```python
from build123d import *

# Parameters (mm, degrees)
PAD_DEPTH   = 25
FILLET_R    = 1.5
FILLET001_R = 1.5


with BuildPart() as part:
    # Sketch → Pad (new body)
    with BuildSketch(Plane.XY):
        with BuildLine():
            Line((0, 0), (0, -45))
            ThreePointArc((-4, -41), (-2.828427, -43.828427), (0, -45))
            Line((-4, -41), (-4, -37))
            ThreePointArc((-4, -37), (-5.171573, -34.171573), (-8, -33))
            Line((-8, -33), (-36, -33))
            ThreePointArc((-40, -29), (-38.828427, -31.828427), (-36, -33))
            Line((-40, -29), (-40, 0))
            ThreePointArc((-36, 0), (-38, 2), (-40, 0))
            Line((-36, 0), (-36, -25))
            ThreePointArc((-36, -25), (-34.828427, -27.828427), (-32, -29))
            Line((-32, -29), (-8, -29))
            ThreePointArc((-8, -29), (-5.171573, -27.828427), (-4, -25))
            Line((-4, -25), (-4, 0))
            ThreePointArc((0, 4), (-2.828427, 2.828427), (-4, 0))
            Line((0, 4), (36, 4))
            ThreePointArc((40, 0), (38.828427, 2.828427), (36, 4))
            Line((40, 0), (0, 0))
        make_face()
    extrude(amount=PAD_DEPTH)

    # Fillet
    fillet_edges = [part.edges().sort_by_distance(p)[0] for p in [
        (-2.828427, -43.828427, 25),
        (-4, -39, 25),
        (-5.171573, -34.171573, 25),
        (-22, -33, 25),
        (-38.828427, -31.828427, 25),
        (-40, -14.5, 25),
        (-38, 2, 25),
        (-36, -12.5, 25),
        (-34.828427, -27.828427, 25),
        (-20, -29, 25),
        (-5.171573, -27.828427, 25),
        (-4, -12.5, 25),
        (-2.828427, 2.828427, 25),
        (18, 4, 25),
        (38.828427, 2.828427, 25),
    ]]
    fillet(fillet_edges, radius=FILLET_R)

    # Fillet001
    fillet001_edges = [part.edges().sort_by_distance(p)[0] for p in [
        (38.828427, 2.828427, 0),
        (18, 4, 0),
        (-2.828427, 2.828427, 0),
        (-4, -12.5, 0),
        (-5.171573, -27.828427, 0),
        (-20, -29, 0),
        (-34.828427, -27.828427, 0),
        (-36, -12.5, 0),
        (-38, 2, 0),
        (-40, -14.5, 0),
        (-38.828427, -31.828427, 0),
        (-22, -33, 0),
        (-5.171573, -34.171573, 0),
        (-4, -39, 0),
        (-2.828427, -43.828427, 0),
    ]]
    fillet(fillet001_edges, radius=FILLET001_R)


solid = part.part
```
Here's how the part is built. I have some questions about the finished solid (model axes, mm). A direction names the side the tool comes from. Coordinates: 2 decimals unless noted, no trailing zeros. Write each loop counter-clockwise with the first axis right and the second up, starting at its lowest first coordinate (ties: lowest second). Pieces come first, ordered by that corner, then holes. Notation, with made-up numbers: (28.25, -28) -> (84.25, -28) arc R23 ccw to (84.25, 9) -> close; hole circle Ø5 at (-1, -7). An arc over 180 degrees is marked (long way). Use a Markdown table: item, result. Add a question column.
(1) We'd pull the mould along X, two halves only. Please class faces 6 (the cylindrical face through (-38.859, -31.797, 12.346)), 7 (the cylindrical face through (-3.55, -12.68, 0.43)), 8 (the cylindrical face through (-21.8, -32.57, 24.55)): +X half, -X half, draft (parallel to the pull), parting line (faces both ways), or undercut.
(2) If we section it at C-C, the plane z = 14.5: Write out the boundary of the cut face in (x, y).
(3) If we section it at A-A, the plane y = -6: Write out the boundary of the cut face in (x, z), and give its area (3 significant figures).
(4) Please list where these lines run through material, in increasing order: line 1 (X direction, y = -17, z = 18); line 2 (Y direction, x = 2, z = 1.75); line 3 (Y direction, x = -19, z = 5.5).
(5) I'm going to push flat-ended pins straight in: P1, Ø4, axis at x = -31.5, z = 15, coming from the -Y side; P2, Ø10, axis at x = -11, z = 17, coming from the +Y side; P3, Ø4, axis at y = -3, z = 13.5, coming from the +X side. Where does each tip first touch, or does it pass through?
(6) If we section it at B-B, the plane x = 22.5: Write out the boundary of the cut face in (y, z), and give its area (3 significant figures).
(7) For faces 1 (the flat face through (6, 2, 0)), 2 (the cylindrical face through (-36.43, -12.32, 24.55)), 3 (the flat face through (-36, -12, 12)), 4 (the cylindrical face through (-36.45, -12.32, 0.43)), 5 (the cylindrical face through (-3.57, -39.03, 24.55)), which set-ups out of +Z, -Z, +X, -X, +Y, -Y let a thin tool reach every point of the face, with its end or its side?
Outcome:
| question | item | result |
|---|---|---|
| 1 | face 6 | -X half |
| 1 | face 7 | undercut |
| 1 | face 8 | draft |
| 2 | outline | (-40, -29) arc R4 ccw to (-36, -33) -> (-8, -33) arc R4 cw to (-4, -37) -> (-4, -41) arc R4 ccw to (0, -45) -> (0, 0) -> (40, 0) arc R4 ccw to (36, 4) -> (0, 4) arc R4 ccw to (-4, 0) -> (-4, -25) arc R4 cw to (-8, -29) -> (-32, -29) arc R4 cw to (-36, -25) -> (-36, 0) arc R2 ccw to (-40, 0) -> close |
| 3 | outline | (-40, 1.5) arc R1.5 ccw to (-38.5, 0) -> (-37.5, 0) arc R1.5 ccw to (-36, 1.5) -> (-36, 23.5) arc R1.5 ccw to (-37.5, 25) -> (-38.5, 25) arc R1.5 ccw to (-40, 23.5) -> close; (-4, 1.5) arc R1.5 ccw to (-2.5, 0) -> (0, 0) -> (0, 25) -> (-2.5, 25) arc R1.5 ccw to (-4, 23.5) -> close |
| 3 | area | 197 mm^2 |
| 4 | line 1 | x = -40 to -36, -4 to 0 |
| 4 | line 2 | y = 0 to 4 |
| 4 | line 3 | y = -33 to -29 |
| 5 | P1 | stops at y = -33 |
| 5 | P2 | stops at y = -28.46 |
| 5 | P3 | stops at x = 0 |
| 6 | outline | (0, 0) -> (2.5, 0) arc R1.5 ccw to (4, 1.5) -> (4, 23.5) arc R1.5 ccw to (2.5, 25) -> (0, 25) -> close |
| 6 | area | 99.0 mm^2 |
| 7 | face 1 | -Z, +X, -X, +Y, -Y |
| 7 | face 2 | +Z, +Y |
| 7 | face 3 | +Z, -Z, +Y |
| 7 | face 4 | -Z, +Y |
| 7 | face 5 | +Z, -X, -Y |
